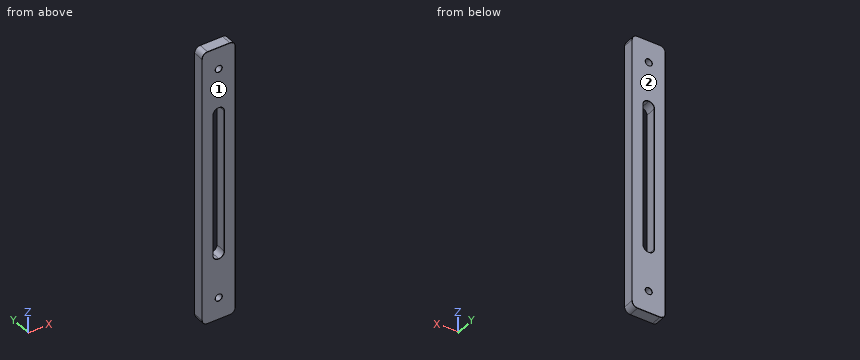
```python
from build123d import *

# Parameters (mm, degrees)
F0_W     = 30
F0_H     = 252
F1_DEPTH = 10
F2_R     = 5
F4_DEPTH = 25
F5_R     = 4.99999
F6_R     = 3
F7_DEPTH = 25
F8_R     = 3
F9_DEPTH = 25
F10_SIZE = 0.2
F11_SIZE = 0.2


# Not quite as in the source:
# - a fillet or chamfer is up to 0.001 mm smaller than in the source, because OpenCascade refuses the exact size


with BuildPart() as f1:
    # F0 (on Front) → F1 (new body)
    with BuildSketch(Plane.XZ):
        with Locations((15, 126)):
            Rectangle(F0_W, F0_H)
    extrude(amount=F1_DEPTH)

    # F2
    f2_edges = [f1.edges().sort_by_distance(p)[0] for p in [
        (30, -5, 252),
        (0, -5, 252),
        (30, -5, 0),
        (0, -5, 0),
    ]]
    fillet(f2_edges, radius=F2_R)

    # F3 (on face) → F4 (cut)
    with BuildSketch(Plane.XZ.offset(10)):
        Polygon((10.0000001118, 196), (10.0000001118, 126), (10.0000001118, 56), (20, 56), (20, 126), (20, 196), align=None)
    extrude(amount=-F4_DEPTH, mode=Mode.SUBTRACT)

    # F5 (radius 5 in the source; OpenCascade refuses exactly that, so slightly less here)
    f5_edges = [f1.edges().sort_by_distance(p)[0] for p in [
        (10, -5, 196),
        (20, -5, 196),
        (20, -5, 56),
        (10, -5, 56),
    ]]
    fillet(f5_edges, radius=F5_R)

    # F6 (on face) → F7 (cut)
    with BuildSketch(Plane.XZ.offset(10)):
        with Locations((15, 232)):
            Circle(F6_R)
    extrude(amount=-F7_DEPTH, mode=Mode.SUBTRACT)

    # F8 (on face) → F9 (cut)
    with BuildSketch(Plane.XZ.offset(10)):
        with Locations((15, 20)):
            Circle(F8_R)
    extrude(amount=-F9_DEPTH, mode=Mode.SUBTRACT)

    # F10
    f10_edges = [f1.edges().sort_by_distance(p)[0] for p in [
        (0, -10, 126),
        (1.464466, -10, 250.535534),
        (1.464466, -10, 1.464466),
        (15, -10, 252),
        (15, -10, 0),
        (28.535534, -10, 250.535534),
        (28.535534, -10, 1.464466),
        (30, -10, 126),
        (12, -10, 20),
        (12, -10, 232),
        (15, -10, 56),
        (11.464463, -10, 57.464463),
        (18.535537, -10, 57.464463),
        (10, -10, 126),
        (20, -10, 126),
        (11.464463, -10, 194.535537),
        (18.535537, -10, 194.535537),
        (15, -10, 196),
    ]]
    chamfer(f10_edges, length=F10_SIZE)

    # F11
    f11_edges = [f1.edges().sort_by_distance(p)[0] for p in [
        (0, 0, 126),
        (1.464466, 0, 250.535534),
        (1.464466, 0, 1.464466),
        (15, 0, 252),
        (15, 0, 0),
        (28.535534, 0, 250.535534),
        (28.535534, 0, 1.464466),
        (30, 0, 126),
        (12, 0, 20),
        (12, 0, 232),
        (10, 0, 126),
        (11.464463, 0, 194.535537),
        (11.464463, 0, 57.464463),
        (15, 0, 196),
        (15, 0, 56),
        (18.535537, 0, 194.535537),
        (18.535537, 0, 57.464463),
        (20, 0, 126),
    ]]
    chamfer(f11_edges, length=F11_SIZE)


solid = f1.part
```
Source: CAD feature listing. Evaluate the final solid. Frame: model axes, mm. Face numbers are marked on the shaded views. Round coordinates to 2 decimals unless told otherwise and drop trailing zeros. Loops run counter-clockwise (first coordinate to the right, second up) from the corner with the lowest first, then second, coordinate; pieces in that order, holes last. Notation, with made-up numbers: M 87,87 L 100,87 A18 cw 100,98 Z; hole C 23.5,85 d1. An arc over 180 degrees is marked long. Put each result on its own line as item: value.
(1) First-contact query: pin 1 (5.5 mm diameter, centred on x = 15, z = 20, fed in from +Y); pin 2 (10 mm diameter, centred on x = 17.5, z = 138, fed in from -Y). Flat tips, straight axial feed; report the tip coordinate or a pass-through.
Solutions:
pin 1: through
pin 2: y = -10
(2) Section C-C, the plane z = 169. Return loops of the section in (x, y), and give its area (3 significant figures).
Solutions:
outline: M 0,-9.8 L 0.2,-10 L 9.8,-10 L 10,-9.8 L 10,-0.2 L 9.8,0 L 0.2,0 L 0,-0.2 Z; M 20,-9.8 L 20.2,-10 L 29.8,-10 L 30,-9.8 L 30,-0.2 L 29.8,0 L 20.2,0 L 20,-0.2 Z
area: 200 mm²
(3) Pull-direction query (Y, two-part tool) for the marked faces 1 and 2; classes: released by +Y, released by -Y, zero draft, split by the parting line, or undercut.
Solutions:
face 1: released by -Y
face 2: released by +Y
(4) Section A-A, the plane z = 232. Return loops of the section in (x, y).
Solutions:
outline: M 0,-9.8 L 0.2,-10 L 11.8,-10 L 12,-9.8 L 12,-0.2 L 11.8,0 L 0.2,0 L 0,-0.2 Z; M 18,-9.8 L 18.2,-10 L 29.8,-10 L 30,-9.8 L 30,-0.2 L 29.8,0 L 18.2,0 L 18,-0.2 Z
(5) Section B-B, the plane y = -7.5. State how many separate pieces and enclosed holes the cut face has, and give its area (3 significant figures).
Solutions:
separate pieces: 1
enclosed holes: 3
area: 6,100 mm²
(6) Ray query, line 1 (X direction, y = -8.5, z = 75.5); line 2 (Z direction, x = 15.5, y = -9); line 3 (X direction, y = -3.5, z = 232). Return the intervals inside material, ascending. Write a range as [from, to].
Solutions:
line 1: [0, 10], [20, 30]
line 2: [0, 17.04], [22.96, 56.03], [195.97, 229.04], [234.96, 252]
line 3: [0, 12], [18, 30]
